Geometry check sheet. Reference: the model listing, model coordinates, mm. Give positions to 0.01 mm unless a question says otherwise; leave off trailing zeros. Loops run counter-clockwise (first coordinate to the right, second up) from the corner with the lowest first, then second, coordinate; pieces in that order, holes last. Notation, with made-up numbers: (16.25, 75) -> (26.25, 75) arc R12 cw to (26.25, 89) -> close; hole circle Ø7 at (-23, 89). An arc over 180 degrees is marked (long way). Write each question's results on one line, items separated by ' | '. Start each with the question number.
1) Scan line: line 1 (X direction, y = -3, z = -2.5). Record every from-to range of solid material in increasing order. Write a range as from..to.
2) Sectioned sample at A-A on z = 3.5. Record the cut outline in (x, y).
```python
from build123d import *

# Parameters (mm, degrees)
ESBO_O1_W                = 10
ESBO_O1_H                = 10
RESSALTO_EXTRUS_O1_DEPTH = 5
CASCA2_T                 = 1
CHANFRO1_SIZE            = 1


with BuildPart() as part:
    # Esboço1 → Ressalto-extrusão1 (new, symmetric)
    with BuildSketch(Plane(origin=(0, 0, 0), x_dir=(1, 0, 0), z_dir=(0, 1, 0))):
        Rectangle(ESBO_O1_W, ESBO_O1_H)
    extrude(amount=RESSALTO_EXTRUS_O1_DEPTH, both=True)

    # Casca2 (no face opened: a closed hollow body)
    add(offset(amount=-CASCA2_T, mode=Mode.PRIVATE), mode=Mode.SUBTRACT)

    # Chanfro1
    chanfro1_edges = [part.edges().sort_by_distance(p)[0] for p in [
        (-5, 5, 0),
        (0, 5, 5),
        (5, 5, 0),
        (0, -5, 5),
        (-5, -5, 0),
        (0, -5, -5),
        (5, -5, 0),
        (5, 0, 5),
        (-5, 0, 5),
        (-5, 0, -5),
        (5, 0, -5),
        (0, 5, -5),
    ]]
    chamfer(chanfro1_edges, length=CHANFRO1_SIZE)


solid = part.part
```
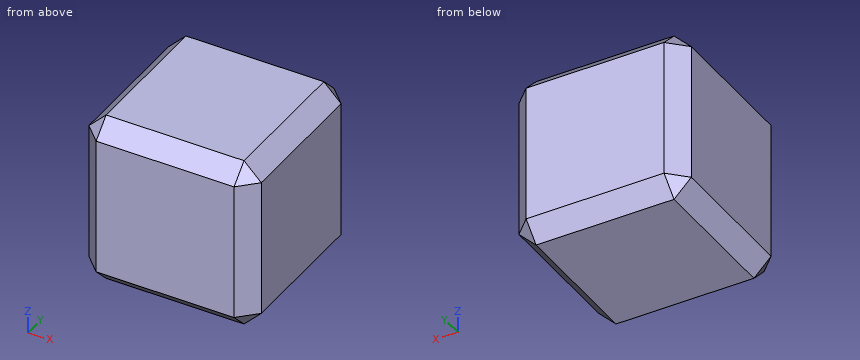
Result:
1) line 1: -5..-4, 4..5
2) outline: (-5, -4) -> (-4, -5) -> (4, -5) -> (5, -4) -> (5, 4) -> (4, 5) -> (-4, 5) -> (-5, 4) -> close; hole (-4, -4) -> (4, -4) -> (4, 4) -> (-4, 4) -> close
